from build123d import *

# Parameters (mm, degrees)
SKETCH1_W           = 3.048
SKETCH1_H           = 6.35
SKETCH1_W_2         = 6.35
SKETCH1_H_2         = 3.048
SKETCH1_W_3         = 5.9944
SKETCH1_H_3         = 5.9944
BOSS_EXTRUDE1_DEPTH = 5.9944


with BuildPart() as part:
    # Sketch1 → Boss-Extrude1 (new body)
    with BuildSketch(Plane(origin=(0, 0, 0), x_dir=(1, 0, 0), z_dir=(0, 1, 0))):
        Polygon((130.175, 0), (130.175, 130.175), (0, 130.175), (0, 168.275), (130.175, 168.275), (130.175, 298.45), (168.275, 298.45), (168.275, 168.275), (298.45, 168.275), (298.45, 130.175), (168.275, 130.175), (168.275, 0), align=None)
        with Locations((163.957, 9.525)):
            Rectangle(SKETCH1_W, SKETCH1_H, mode=Mode.SUBTRACT)
        with Locations((134.493, 9.525)):
            Rectangle(SKETCH1_W, SKETCH1_H, mode=Mode.SUBTRACT)
        with Locations((288.925, 163.957)):
            Rectangle(SKETCH1_W_2, SKETCH1_H_2, mode=Mode.SUBTRACT)
        with Locations((288.925, 134.493)):
            Rectangle(SKETCH1_W_2, SKETCH1_H_2, mode=Mode.SUBTRACT)
        with Locations((149.225, 196.723)):
            Rectangle(SKETCH1_W, SKETCH1_H, mode=Mode.SUBTRACT)
        with Locations((101.727, 149.225)):
            Rectangle(SKETCH1_W_2, SKETCH1_H_2, mode=Mode.SUBTRACT)
        with Locations((149.225, 163.449)):
            Rectangle(SKETCH1_W_2, SKETCH1_H_2, mode=Mode.SUBTRACT)
        with Locations((135.001, 149.225)):
            Rectangle(SKETCH1_W, SKETCH1_H, mode=Mode.SUBTRACT)
        with Locations((163.449, 149.225)):
            Rectangle(SKETCH1_W, SKETCH1_H, mode=Mode.SUBTRACT)
        with Locations((196.723, 149.225)):
            Rectangle(SKETCH1_W_2, SKETCH1_H_2, mode=Mode.SUBTRACT)
        with Locations((149.225, 135.001)):
            Rectangle(SKETCH1_W_2, SKETCH1_H_2, mode=Mode.SUBTRACT)
        with Locations((149.225, 101.727)):
            Rectangle(SKETCH1_W, SKETCH1_H, mode=Mode.SUBTRACT)
        with Locations((134.493, 66.3194)):
            Rectangle(SKETCH1_W, SKETCH1_H, mode=Mode.SUBTRACT)
        with Locations((163.957, 66.3194)):
            Rectangle(SKETCH1_W, SKETCH1_H, mode=Mode.SUBTRACT)
        with Locations((232.1306, 134.493)):
            Rectangle(SKETCH1_W_2, SKETCH1_H_2, mode=Mode.SUBTRACT)
        with Locations((232.1306, 163.957)):
            Rectangle(SKETCH1_W_2, SKETCH1_H_2, mode=Mode.SUBTRACT)
        with Locations((260.5278, 149.225)):
            Rectangle(SKETCH1_W_3, SKETCH1_H, mode=Mode.SUBTRACT)
        with Locations((149.225, 37.9222)):
            Rectangle(SKETCH1_W_2, SKETCH1_H_3, mode=Mode.SUBTRACT)
        with Locations((149.225, 260.5278)):
            Rectangle(SKETCH1_W_2, SKETCH1_H_3, mode=Mode.SUBTRACT)
        with Locations((163.957, 232.1306)):
            Rectangle(SKETCH1_W, SKETCH1_H, mode=Mode.SUBTRACT)
        with Locations((134.493, 232.1306)):
            Rectangle(SKETCH1_W, SKETCH1_H, mode=Mode.SUBTRACT)
        with Locations((134.493, 288.925)):
            Rectangle(SKETCH1_W, SKETCH1_H, mode=Mode.SUBTRACT)
        with Locations((163.957, 288.925)):
            Rectangle(SKETCH1_W, SKETCH1_H, mode=Mode.SUBTRACT)
        with Locations((37.9222, 149.225)):
            Rectangle(SKETCH1_W_3, SKETCH1_H, mode=Mode.SUBTRACT)
        with Locations((66.3194, 163.957)):
            Rectangle(SKETCH1_W_2, SKETCH1_H_2, mode=Mode.SUBTRACT)
        with Locations((66.3194, 134.493)):
            Rectangle(SKETCH1_W_2, SKETCH1_H_2, mode=Mode.SUBTRACT)
        with Locations((9.525, 134.493)):
            Rectangle(SKETCH1_W_2, SKETCH1_H_2, mode=Mode.SUBTRACT)
        with Locations((9.525, 163.957)):
            Rectangle(SKETCH1_W_2, SKETCH1_H_2, mode=Mode.SUBTRACT)
    extrude(amount=BOSS_EXTRUDE1_DEPTH)


solid = part.part
Could you check a few things on this model? Use its own coordinates, in mm. Coordinates: 2 decimals unless noted, no trailing zeros. Order: outer loops, then holes, each group sorted by start corner. A loop starts at its lowest first (then second) coordinate and runs counter-clockwise, first axis right, second up. Notation, with made-up numbers: (6.25, 49) -> (11.25, 49) arc R8 ccw to (11.25, 62) -> close; hole circle Ø7 at (7.25, 36). An arc over 180 degrees is marked (long way). One line per item, written item: value. Start each with the question number.
1) I'm going to push flat-ended pins straight in: pin 1 (3 mm diameter, centred on y = 3, z = -230.5, fed in from -X) (3 decimals); pin 2 (1 mm diameter, centred on x = 39.5, y = 1.5, fed in from -Z) (3 decimals). Where does each tip first touch, or does it pass through?
2) Imagine slicing it at B-B on x = 241. List the corners of the cut face in (y, z) for me (3 decimals).
3) Imagine slicing it at C-C on z = -19. List the corners of the cut face in (x, y) for me (3 decimals), plus the area to 3 significant figures.
4) Imagine slicing it at A-A on y = 1.45. Count the separate pieces of the cut face and the enclosed holes in it, plus the area to 3 significant figures.
5) If I drill on L1, parallel to X at y = 2.85, z = -151 (3 decimals); L2, parallel to X at y = 5.05, z = -66 (3 decimals); L3, parallel to Z at x = 194.5, y = 3.9 (3 decimals), over which ranges is the centre line in solid material (lowest first)? Write a range as [from, to].
Answer list:
1. pin 1: stops at x = 130.175
1. pin 2: stops at z = -168.275
2. outline: (0, -168.275) -> (5.994, -168.275) -> (5.994, -130.175) -> (0, -130.175) -> close
3. outline: (130.175, 0) -> (168.275, 0) -> (168.275, 5.994) -> (130.175, 5.994) -> close
3. area: 228 mm2
4. separate pieces: 1
4. enclosed holes: 28
4. area: 20,700 mm2
5. L1: x = [0, 34.925], [40.919, 133.477], [136.525, 161.925], [164.973, 257.531], [263.525, 298.45]
5. L2: x = [130.175, 132.969], [136.017, 162.433], [165.481, 168.275]
5. L3: z = [-168.275, -150.749], [-147.701, -130.175]
